CAD build for the part. Positions are in the model's coordinates, mm. Coordinates: 2 decimals unless noted, no trailing zeros. Write each loop counter-clockwise with the first axis right and the second up, starting at its lowest first coordinate (ties: lowest second). Pieces come first, ordered by that corner, then holes. Notation, with made-up numbers: (13.25, 2) -> (26.25, 2) arc R24 ccw to (26.25, 37) -> close; hole circle Ø3 at (-14, 9). An arc over 180 degrees is marked (long way). Answer as CSV lines item,"result".
```python
from build123d import *

# Parameters (mm, degrees)
SKETCH1_R           = 1.5
BOSS_EXTRUDE1_DEPTH = 10
CUT_EXTRUDE1_DEPTH  = 1.2
SKETCH3_OUTSIDE_W   = 9.572
SKETCH3_OUTSIDE_H   = 9.572
SKETCH3_OUTSIDE_R   = 1.18
CUT_EXTRUDE2_DEPTH  = 1.2
CUT_EXTRUDE2_DRAFT  = -45
SKETCH4_OUTSIDE_W   = 9.572
SKETCH4_OUTSIDE_H   = 9.572
SKETCH4_OUTSIDE_R   = 0.375
CUT_EXTRUDE3_DEPTH  = 1.2
CUT_EXTRUDE3_DRAFT  = -45


with BuildPart() as part:
    # Sketch1 → Boss-Extrude1 (new body)
    with BuildSketch(Plane.XY):
        Circle(SKETCH1_R)
    extrude(amount=BOSS_EXTRUDE1_DEPTH)

    # Sketch2 → Cut-Extrude1 (cut)
    with BuildSketch(Plane.XY.offset(10)):
        Polygon((0.867651504, 0), (0.433825752, 0.751408244), (-0.433825752, 0.751408244), (-0.867651504, 0), (-0.433825752, -0.751408244), (0.433825752, -0.751408244), align=None)
    extrude(amount=-CUT_EXTRUDE1_DEPTH, mode=Mode.SUBTRACT)


with BuildPart() as cut_extrude2_tool:
    # Sketch3 outside → Cut-Extrude2 (with draft: the straight prism first)
    with BuildSketch(Plane.XY.offset(10)):
        Rectangle(SKETCH3_OUTSIDE_W, SKETCH3_OUTSIDE_H)
        Circle(SKETCH3_OUTSIDE_R, mode=Mode.SUBTRACT)
    extrude(amount=-CUT_EXTRUDE2_DEPTH)
    # Cut-Extrude2: the draft: its side faces are tilted about the plane it starts from
    cut_extrude2_sides = [cut_extrude2_tool.faces().sort_by_distance(p)[0] for p in [
        (0, -4.786, 9.4),
        (4.786, 0, 9.4),
        (0, 4.786, 9.4),
        (-4.786, 0, 9.4),
        (-1.18, 0, 9.4),
    ]]
    draft(cut_extrude2_sides, Plane.XY.offset(10), CUT_EXTRUDE2_DRAFT)


with BuildPart() as part_1:
    add(part.part)

    # Cut-Extrude2: cut by cut_extrude2_tool
    add(cut_extrude2_tool.part, mode=Mode.SUBTRACT)


with BuildPart() as cut_extrude3_tool:
    # Sketch4 outside → Cut-Extrude3 (with draft: the straight prism first)
    with BuildSketch(Plane(origin=(0, 0, 0), x_dir=(-1, 0, 0), z_dir=(0, 0, -1))):
        Rectangle(SKETCH4_OUTSIDE_W, SKETCH4_OUTSIDE_H)
        Circle(SKETCH4_OUTSIDE_R, mode=Mode.SUBTRACT)
    extrude(amount=-CUT_EXTRUDE3_DEPTH)
    # Cut-Extrude3: the draft: its side faces are tilted about the plane it starts from
    cut_extrude3_sides = [cut_extrude3_tool.faces().sort_by_distance(p)[0] for p in [
        (0, -4.786, 0.6),
        (-4.786, 0, 0.6),
        (0, 4.786, 0.6),
        (4.786, 0, 0.6),
        (0.375, 0, 0.6),
    ]]
    draft(cut_extrude3_sides, Plane(origin=(0, 0, 0), x_dir=(-1, 0, 0), z_dir=(0, 0, -1)), CUT_EXTRUDE3_DRAFT)


with BuildPart() as part_2:
    add(part_1.part)

    # Cut-Extrude3: cut by cut_extrude3_tool
    add(cut_extrude3_tool.part, mode=Mode.SUBTRACT)


solid = part_2.part
```
Item 1: Saw through at B-B on z = 6.5. Give the cut face in (x, y).
Answer below:
outline,"circle Ø3 at (0, 0)"
Item 2: Two-plate mould, pull along Y, no slides. Class faces 1 (the flat face through (0, 0, 8.8)), 2 (the flat face through (0, -1, 10)), 3 (the cylindrical face through (-1.5, 0.07, 5.34)): pulls with the +Y half, pulls with the -Y half, needs draft (parallel to the pull), parting line crosses it, or undercut.
Answer below:
face 1,"undercut"
face 2,"needs draft"
face 3,"parting line crosses it"
Item 3: Saw through at A-A on x = 0. Give the cut face in (y, z) (3 decimals), and give its area (3 significant figures).
Answer below:
outline,"(-1.5, 1.125) -> (-0.375, 0) -> (0.375, 0) -> (1.5, 1.125) -> (1.5, 9.68) -> (1.18, 10) -> (0.751, 10) -> (0.751, 8.8) -> (-0.751, 8.8) -> (-0.751, 10) -> (-1.18, 10) -> (-1.5, 9.68) -> close"
area,"26.8 mm2"
Item 4: Wall check: line 1 (X direction, y = 0.2, z = 9); line 2 (X direction, y = 0.35, z = 9.75); line 3 (X direction, y = 0.95, z = 7.25). Give the ranges that are in metal, low to high. Write a range as from..to.
Answer below:
line 1,"x = -1.49..-0.75, 0.75..1.49"
line 2,"x = -1.39..-0.67, 0.67..1.39"
line 3,"x = -1.16..1.16"
Item 5: Flat gauge pin, fed straight in: pin 1 (1.2 mm diameter, centred on x = 0, y = 0, fed in from +Z). Where does the tip first touch, or does it go through?
Answer below:
pin 1,"stops at z = 8.8"
